Print and shaded views of the part. All mm, measured from the part's lowest x, y and z. Round coordinates to 2 decimals unless told otherwise and drop trailing zeros. Write each loop counter-clockwise with the first axis right and the second up, starting at its lowest first coordinate (ties: lowest second). Pieces come first, ordered by that corner, then holes. Notation, with made-up numbers: (-24.75, -35.75) - (-12.75, -35.75) arc R23 ccw to (-12.75, -22.75) - close; hole circle Ø1 at (88, -30.75). An arc over 180 degrees is marked (long way). Answer as a JSON object with one key per item and string values. Group by question number.
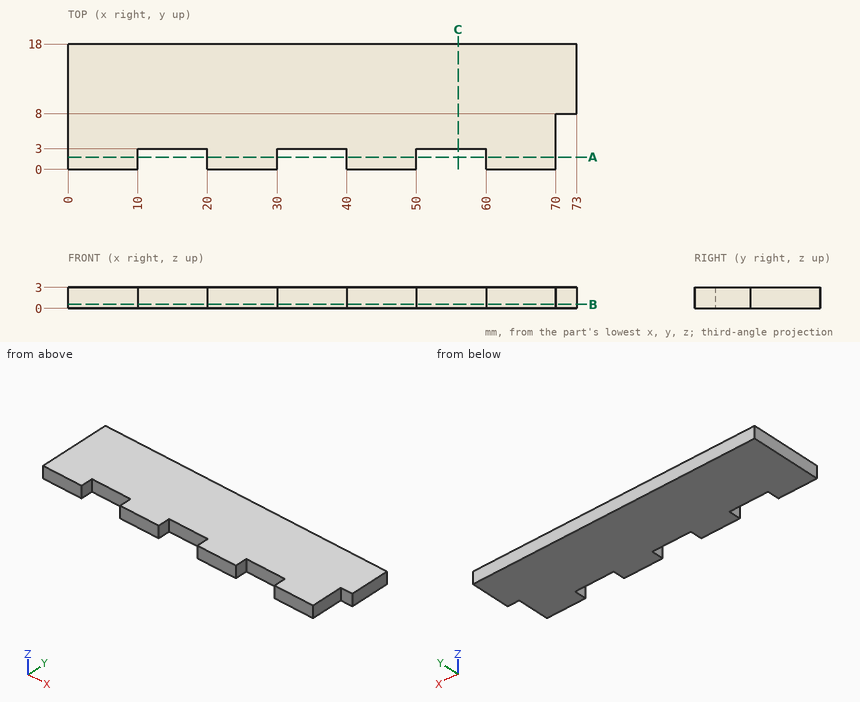
(1) Slice it at A-A (y = 1.75). Write the cut outline in (x, z), then the cut area to 3 significant figures.
(2) Slice it at B-B (z = 0.55). Write the cut outline in (x, y), then the cut area to 3 significant figures.
(3) Drill centre lines: line 1 (Y direction, x = 11, z = 2); line 2 (X direction, y = 6, z = 0.6). Where is each one in solid material? Low to high. Write a range as from..to.
(4) Slice it at C-C (x = 56). Write the cut outline in (y, z), then the cut area to 3 significant figures.
(5) Flat gauge pin, fed straight in: pin 1 (0.9 mm diameter, centred on y = 5, z = 2, fed in from +X). Where does the tip first touch, or does it go through?
Answer:
{
 "1": {"outline": "(0, 0) - (10, 0) - (10, 3) - (0, 3) - close; (20, 0) - (30, 0) - (30, 3) - (20, 3) - close; (40, 0) - (50, 0) - (50, 3) - (40, 3) - close; (60, 0) - (70, 0) - (70, 3) - (60, 3) - close", "area": "120 mm²"},
 "2": {"outline": "(0, 0) - (10, 0) - (10, 3) - (20, 3) - (20, 0) - (30, 0) - (30, 3) - (40, 3) - (40, 0) - (50, 0) - (50, 3) - (60, 3) - (60, 0) - (70, 0) - (70, 8) - (73, 8) - (73, 18) - (0, 18) - close", "area": "1,200 mm²"},
 "3": {"line 1": "3..18", "line 2": "0..70"},
 "4": {"outline": "(3, 0) - (18, 0) - (18, 3) - (3, 3) - close", "area": "45.0 mm²"},
 "5": {"pin 1": "x = 70"}
}
